Source: three-view drawing plus pictorial views. Frame: mm from the lowest corner of the part. Round coordinates to 2 decimals unless told otherwise and drop trailing zeros. Loops run counter-clockwise (first coordinate to the right, second up) from the corner with the lowest first, then second, coordinate; pieces in that order, holes last. Notation, with made-up numbers: M -18.5,37 L -3.5,37 A17 cw -3.5,42 Z; hole C 65.25,21 d9. An arc over 180 degrees is marked long. Answer as a JSON object with one key per item and string values.
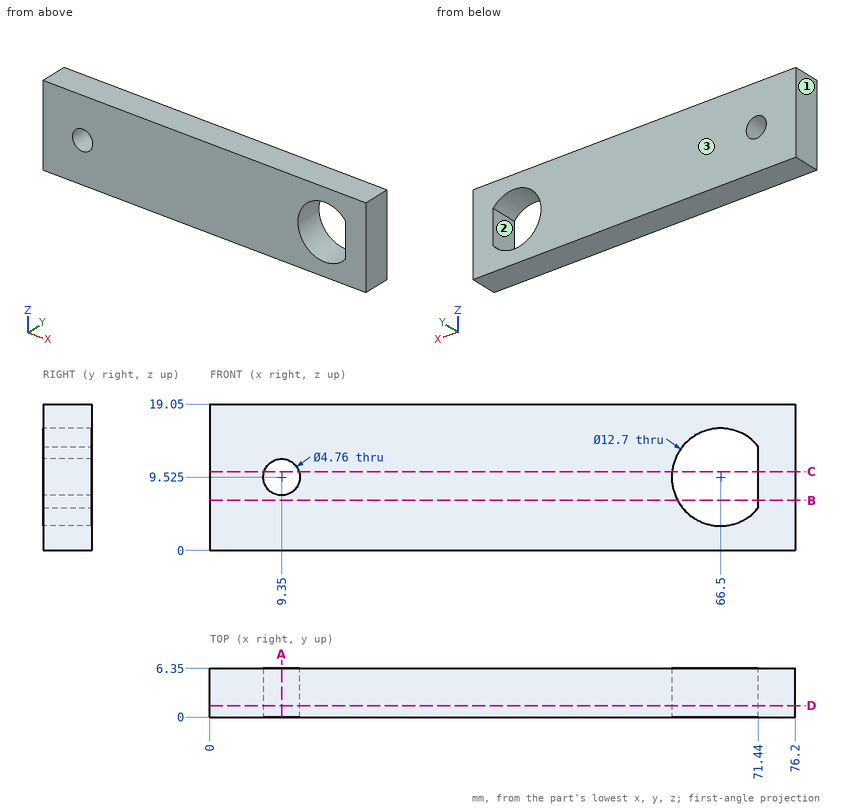
1) Cut plane A-A on x = 9.35. Return the cut outline in (y, z) (3 decimals).
Geometry results:
{"outline": "M 0,0 L 6.35,0 L 6.35,7.145 L 0,7.145 Z; M 0,11.905 L 6.35,11.905 L 6.35,19.05 L 0,19.05 Z"}
2) Cut plane C-C on z = 10.25. Return the cut outline in (x, y), and give its area (3 significant figures).
Geometry results:
{"outline": "M 0,0 L 7.08,0 L 7.08,6.35 L 0,6.35 Z; M 11.62,0 L 60.19,0 L 60.19,6.35 L 11.62,6.35 Z; M 71.44,0 L 76.2,0 L 76.2,6.35 L 71.44,6.35 Z", "area": "384 mm2"}
3) Cut plane B-B on z = 6.5. Return the cut outline in (x, y).
Geometry results:
{"outline": "M 0,0 L 60.92,0 L 60.92,6.35 L 0,6.35 Z; M 71.44,0 L 76.2,0 L 76.2,6.35 L 71.44,6.35 Z"}
4) Pull-direction query (X, two-part tool) for the marked faces 1, 2 and 3; classes: +X half, -X half, draft (parallel to the pull), parting line (faces both ways), or undercut.
Geometry results:
{"face 1": "-X half", "face 2": "undercut", "face 3": "draft"}
5) Line query: probe 1 along Z at (x, y) = (9.35, 2.5) (3 decimals); probe 2 along Z at (x, y) = (66.5, 2) (3 decimals); probe 3 along X at (y, z) = (2, 7.5). Output: solid intervals per line, ascending.
Geometry results:
{"probe 1": "0 to 7.145, 11.905 to 19.05", "probe 2": "0 to 3.175, 15.875 to 19.05", "probe 3": "0 to 8.1, 10.6 to 60.48, 71.44 to 76.2"}
6) Cut plane D-D on y = 1.5. Return the cut outline in (x, z) (3 decimals), and give its area (3 significant figures).
Geometry results:
{"outline": "M 0,0 L 76.2,0 L 76.2,19.05 L 0,19.05 Z; hole C 9.35,9.525 d4.76; hole M 71.44,5.535 L 71.44,13.515 A6.35 ccw long Z", "area": "1,310 mm2"}
